from build123d import *

# Parameters (mm, degrees)
SZKIC1_R                    = 2.5
DODANIE_WYCI_GNI_CIE1_DEPTH = 1.35
SZKIC2_OUTSIDE_W            = 21.856
SZKIC2_OUTSIDE_H            = 23.094
SZKIC2_OUTSIDE_R            = 4
WYTNIJ_WYCI_GNI_CIE2_DEPTH  = 2.7
WYTNIJ_WYCI_GNI_CIE2_DRAFT  = -60
LUSTRO1_COPY_1_SKETCH_W     = 21.856
LUSTRO1_COPY_1_SKETCH_H     = 23.094
LUSTRO1_COPY_1_SKETCH_R     = 4
LUSTRO1_COPY_1_DEPTH        = 2.7
LUSTRO1_COPY_1_DRAFT        = -60


with BuildPart() as part:
    # Szkic1 → Dodanie-wyciągnięcie1 (new, symmetric)
    with BuildSketch(Plane.XY):
        Polygon((-4, 2.309401077), (-4, -2.309401077), (0, -4.618802154), (4, -2.309401077), (4, 2.309401077), (0, 4.618802154), align=None)
        with Locations(Location((0, 0, 0), (0, 0, 180))):
            Circle(SZKIC1_R, mode=Mode.SUBTRACT)
    extrude(amount=DODANIE_WYCI_GNI_CIE1_DEPTH, both=True)


with BuildPart() as wytnij_wyci_gni_cie2_tool:
    # Szkic2 outside → Wytnij-wyciągnięcie2 (with draft: the straight prism first)
    with BuildSketch(Plane.XY.offset(1.35)):
        Rectangle(SZKIC2_OUTSIDE_W, SZKIC2_OUTSIDE_H)
        Circle(SZKIC2_OUTSIDE_R, mode=Mode.SUBTRACT)
    extrude(amount=-WYTNIJ_WYCI_GNI_CIE2_DEPTH)
    # Wytnij-wyciągnięcie2: the draft: its side faces are tilted about the plane it starts from
    wytnij_wyci_gni_cie2_sides = [wytnij_wyci_gni_cie2_tool.faces().sort_by_distance(p)[0] for p in [
        (0, -11.547, 0),
        (10.928, 0, 0),
        (0, 11.547, 0),
        (-10.928, 0, 0),
        (-4, 0, 0),
    ]]
    draft(wytnij_wyci_gni_cie2_sides, Plane.XY.offset(1.35), WYTNIJ_WYCI_GNI_CIE2_DRAFT)


with BuildPart() as part_1:
    add(part.part)

    # Wytnij-wyciągnięcie2: cut by wytnij_wyci_gni_cie2_tool
    add(wytnij_wyci_gni_cie2_tool.part, mode=Mode.SUBTRACT)


with BuildPart() as lustro1_copy_1_tool:
    # Lustro1 copy 1 sketch → Lustro1 copy 1 (with draft: the straight prism first)
    with BuildSketch(Plane(origin=(0, 0, -1.35), x_dir=(1, 0, 0), z_dir=(0, 0, -1))):
        Rectangle(LUSTRO1_COPY_1_SKETCH_W, LUSTRO1_COPY_1_SKETCH_H)
        Circle(LUSTRO1_COPY_1_SKETCH_R, mode=Mode.SUBTRACT)
    extrude(amount=-LUSTRO1_COPY_1_DEPTH)
    # Lustro1 copy 1: the draft: its side faces are tilted about the plane it starts from
    lustro1_copy_1_sides = [lustro1_copy_1_tool.faces().sort_by_distance(p)[0] for p in [
        (0, -11.547, 0),
        (10.928, 0, 0),
        (0, 11.547, 0),
        (-10.928, 0, 0),
        (-4, 0, 0),
    ]]
    draft(lustro1_copy_1_sides, Plane(origin=(0, 0, -1.35), x_dir=(1, 0, 0), z_dir=(0, 0, -1)), LUSTRO1_COPY_1_DRAFT)


with BuildPart() as part_2:
    add(part_1.part)

    # Lustro1 copy 1: cut by lustro1_copy_1_tool
    add(lustro1_copy_1_tool.part, mode=Mode.SUBTRACT)


solid = part_2.part
Model file for the job. Use its own axes, mm. Give positions to 0.01 mm unless a question says otherwise; leave off trailing zeros. Order: outer loops, then holes, each group sorted by start corner. A loop starts at its lowest first (then second) coordinate and runs counter-clockwise, first axis right, second up. Notation, with made-up numbers: (75.5, -33.75) - (109.5, -33.75) arc R20 ccw to (109.5, -16.75) - close; hole circle Ø6 at (59, -36). An arc over 180 degrees is marked (long way). Return JSON: item names as keys, results as strings.
1) Flat gauge pin, fed straight in: P1, Ø1.5, axis at y = -3.5, z = -0.5, coming from the +X side. Where does the tip first touch, or does it go through?
Geometry says:
{"P1": "x = 3.24"}
2) Cut at A-A, the plane z = -0.15. Give the cut face in (x, y), plus the area to 3 significant figures.
Geometry says:
{"outline": "(-4, -2.31) - (0, -4.62) - (4, -2.31) - (4, 2.31) - (0, 4.62) - (-4, 2.31) - close; hole circle Ø5 at (0, 0)", "area": "35.8 mm²"}
3) Pull direction X, two halves, no side cores. Call faces 1 (the conical face through (-3.587, 2.083, 1.265)), 2 (the flat face through (2, 2, 1.35)), 3 (the cylindrical face through (2.5, -0.1, 0)): pulls with the +X half, pulls with the -X half, needs draft (parallel to the pull), parting line crosses it, or undercut.
Geometry says:
{"face 1": "pulls with the -X half", "face 2": "needs draft", "face 3": "undercut"}
4) Probe line 1 (X direction, y = 1.5, z = 0.05); line 2 (X direction, y = 2, z = 0.5); line 3 (Y direction, x = 0.5, z = 0.25). List the from-to ranges inside material, lowest first. Write a range as from..to.
Geometry says:
{"line 1": "-4..-2, 2..4", "line 2": "-4..-1.5, 1.5..4", "line 3": "-4.33..-2.45, 2.45..4.33"}
